Geometry check sheet. Reference: the model listing, model coordinates, mm. A direction names the side the tool comes from. Round coordinates to 2 decimals unless told otherwise and drop trailing zeros. Loops run counter-clockwise (first coordinate to the right, second up) from the corner with the lowest first, then second, coordinate; pieces in that order, holes last. Notation, with made-up numbers: (-19.75, 75.25) - (29.25, 75.25) arc R10 ccw to (29.25, 86.25) - close; hole circle Ø3 at (21.25, -2). An arc over 180 degrees is marked (long way). Write item = value, one per line.
```python
from build123d import *

# Parameters (mm, degrees)
SKETCH1_R                            = 10
BOSS_EXTRUDE1_DEPTH                  = 10
SKETCH1_R_2                          = 20
SKETCH1_R_3                          = 15
BOSS_EXTRUDE1_2_DEPTH                = 10
SKETCH1_R_4                          = 40
SKETCH1_R_5                          = 35
BOSS_EXTRUDE1_3_DEPTH                = 10
BOSS_EXTRUDE2_REACH                  = 89.446
BOSS_EXTRUDE2_END_RADIUS             = 35
BOSS_EXTRUDE2_START                  = 30
BOSS_EXTRUDE2_DIRECTION_2_REACH      = 89.446
BOSS_EXTRUDE2_DIRECTION_2_END_RADIUS = 20
CIRPATTERN1_COUNT                    = 12
BOSS_EXTRUDE3_START                  = 9.76079
BOSS_EXTRUDE3_DEPTH                  = 5.23921
CIRPATTERN3_COUNT                    = 3
SKETCH6_R                            = 1
BOSS_EXTRUDE4_DEPTH                  = 1


with BuildPart() as part:
    # Sketch1 → Boss-Extrude1 (new body)
    with BuildSketch(Plane(origin=(0, 0, 0), x_dir=(1, 0, 0), z_dir=(0, 1, 0))):
        with Locations(Location((0, 0, 0), (0, 0, 270))):
            Circle(SKETCH1_R)
    extrude(amount=BOSS_EXTRUDE1_DEPTH)



with BuildPart() as body_2:
    # Sketch1 → Boss-Extrude1 2 (new body)
    with BuildSketch(Plane(origin=(0, 0, 0), x_dir=(1, 0, 0), z_dir=(0, 1, 0))):
        with Locations(Location((0, 0, 0), (0, 0, 270))):
            Circle(SKETCH1_R_2)
        with Locations(Location((0, 0, 0), (0, 0, 270))):
            Circle(SKETCH1_R_3, mode=Mode.SUBTRACT)
    extrude(amount=BOSS_EXTRUDE1_2_DEPTH)


with BuildPart() as body_3:
    # Sketch1 → Boss-Extrude1 3 (new body)
    with BuildSketch(Plane(origin=(0, 0, 0), x_dir=(1, 0, 0), z_dir=(0, 1, 0))):
        with Locations(Location((0, 0, 0), (0, 0, 270))):
            Circle(SKETCH1_R_4)
        with Locations(Location((0, 0, 0), (0, 0, 270))):
            Circle(SKETCH1_R_5, mode=Mode.SUBTRACT)
    extrude(amount=BOSS_EXTRUDE1_3_DEPTH)


    add(body_2.part)  # Boss-Extrude2 merges body 2
    # Boss-Extrude2: up to this cylinder (the profile starts inside it)
    boss_extrude2_end = Plane(origin=(0, 5, 0), z_dir=(0, -1, 0)) * Cylinder(BOSS_EXTRUDE2_END_RADIUS, 249.892, mode=Mode.PRIVATE)
    # Sketch4 → Boss-Extrude2 (add, up to the surface)
    with BuildSketch(Plane(origin=(0, 0, 0), x_dir=(0, 0, -1), z_dir=(1, 0, 0)).offset(BOSS_EXTRUDE2_START), mode=Mode.PRIVATE) as boss_extrude2_sk1:
        Polygon((-4.262410526, 0), (4.031443844, 10), (5.315133993, 10), (-2.978720377, 0), align=None)
    boss_extrude2_tool1 = extrude(boss_extrude2_sk1.sketch, amount=BOSS_EXTRUDE2_REACH, mode=Mode.PRIVATE) & boss_extrude2_end
    boss_extrude2 = boss_extrude2_tool1.solids().sort_by_distance((30, 5, -0.526362))[0]
    add(boss_extrude2)

    # Boss-Extrude2 direction 2: up to this cylinder (the profile starts outside it)
    boss_extrude2_direction_2_end = Plane(origin=(0, 5, 0), z_dir=(0, -1, 0)) * Cylinder(BOSS_EXTRUDE2_DIRECTION_2_END_RADIUS, 219.892, mode=Mode.PRIVATE)
    # Sketch4 → Boss-Extrude2 direction 2 (add, up to the surface)
    with BuildSketch(Plane(origin=(0, 0, 0), x_dir=(0, 0, -1), z_dir=(1, 0, 0)).offset(BOSS_EXTRUDE2_START), mode=Mode.PRIVATE) as boss_extrude2_direction_2_sk1:
        Polygon((-4.262410526, 0), (4.031443844, 10), (5.315133993, 10), (-2.978720377, 0), align=None)
    boss_extrude2_direction_2_tool1 = extrude(boss_extrude2_direction_2_sk1.sketch, amount=-BOSS_EXTRUDE2_DIRECTION_2_REACH, mode=Mode.PRIVATE) - boss_extrude2_direction_2_end
    boss_extrude2_direction_2 = boss_extrude2_direction_2_tool1.solids().sort_by_distance((30, 5, -0.526362))[0]
    add(boss_extrude2_direction_2)
    boss_extrude2 = boss_extrude2 + boss_extrude2_direction_2  # both directions under the feature's name, for the pattern or mirror that repeats it

    # CirPattern1: Boss-Extrude2 ×12 about axis
    cirpattern1_axis = Axis((0, 0, 0), (0, 1, 0))
    for i in range(1, CIRPATTERN1_COUNT):
        add(boss_extrude2.rotate(cirpattern1_axis, i * 360 / CIRPATTERN1_COUNT))


with BuildPart() as part_1:
    add(part.part)

    add(body_3.part)  # Boss-Extrude3 merges body 3
    # Sketch5 → Boss-Extrude3 (add)
    with BuildSketch(Plane(origin=(0, 0, 0), x_dir=(0, 0, -1), z_dir=(1, 0, 0)).offset(BOSS_EXTRUDE3_START)):
        Polygon((-2.0524403, 10), (1.416675924, 0), (2.174160553, 0), (-1.428789261, 10), align=None)
    boss_extrude3 = extrude(amount=BOSS_EXTRUDE3_DEPTH)

    # CirPattern3: Boss-Extrude3 ×3 about axis
    cirpattern3_axis = Axis((0, 0, 0), (0, 1, 0))
    for i in range(1, CIRPATTERN3_COUNT):
        add(boss_extrude3.rotate(cirpattern3_axis, i * 360 / CIRPATTERN3_COUNT))

    # Sketch6 → Boss-Extrude4 (add)
    with BuildSketch(Plane(origin=(0, 10, 0), x_dir=(1, 0, 0), z_dir=(0, 1, 0))):
        with Locations(Location((0, 0, 0), (0, 0, 270))):
            Circle(SKETCH6_R)
    extrude(amount=BOSS_EXTRUDE4_DEPTH)


solid = part_1.part
```
(1) Mould release check, pull along X, two halves, no side actions. Record for faces 1 (the flat face through (22.8, 5.07, -14.58)), 2 (the flat face through (-8, 10, -1)), 3 (the flat face through (-5.88, 5.07, -10.87)), 4 (the cylindrical face through (-0.976, 10.493, -0.217)): pulls with the +X half, pulls with the -X half, needs draft (parallel to the pull), parting line crosses it, or undercut.
Answers follow:
face_1 = undercut
face_2 = needs draft
face_3 = undercut
face_4 = parting line crosses it
(2) Section check B-B (x = 0). State how many separate pieces and enclosed holes the cut face has, then the cut area to 3 significant figures.
Answers follow:
separate_pieces = 3
enclosed_holes = 0
area = 448 mm²
(3) Section check A-A (x = 11). Enter the section's corners in (y, z), then the cut area to 3 significant figures.
Answers follow:
outline = (0, -38.46) - (10, -38.46) - (10, -33.23) - (0, -33.23) - close; (0, -16.7) - (2.18, -16.7) - (10, -29.68) - (10, -27.12) - (3.72, -16.7) - (10, -16.7) - (10, -10.2) - (0, -10.2) - close; (0, -2.17) - (10, 1.43) - (10, 2.05) - (0, -1.42) - close; (0, 10.2) - (10, 10.2) - (10, 16.7) - (6.56, 16.7) - (0, 27.58) - (0, 25.01) - (5.01, 16.7) - (0, 16.7) - close; (0, 33.23) - (10, 33.23) - (10, 38.46) - (0, 38.46) - close
area = 275 mm²
(4) Gauge pin test, flat ends, axial feed: pin 1 (1.5 mm diameter, centred on x = 10, y = 2, fed in from +Z); pin 2 (2 mm diameter, centred on y = 2, z = -29, fed in from +X); pin 3 (6 mm diameter, centred on x = 22, z = -7, fed in from +Y). Record the tip position at first contact, or that the pin passes through.
Answers follow:
pin_1 = 38.92
pin_2 = 28.57
pin_3 = 10
(5) Set-up check for faces 5 (the flat face through (-6.475, 5.07, 10.53)), 6 (the cylindrical face through (-9.398, 4.93, -33.715)), 7 (the flat face through (-5.83, 4.93, 10.89)): record each of +Z, -Z, +X, -X, +Y, -Y from which the full face is reachable in a straight line by a thin tool's end or side.
Answers follow:
face_5 = -Y
face_6 = none
face_7 = +Y
(6) Section check D-D (x = 25.5). Enter the section's corners in (y, z).
Answers follow:
outline = (0, -30.82) - (10, -30.82) - (10, -23.97) - (0, -23.97) - close; (0, -11.28) - (10, -20.86) - (10, -19.38) - (0, -9.8) - close; (0, 2.98) - (10, -5.32) - (10, -4.03) - (0, 4.26) - close; (0, 18.16) - (10, 8.59) - (10, 10.07) - (0, 19.64) - close; (0, 23.97) - (10, 23.97) - (10, 30.82) - (0, 30.82) - close
(7) Scan lines: L1, parallel to Z at x = 0.5, y = 8; L2, parallel to Z at x = -17, y = 5.25; L3, parallel to X at y = 5.75, z = 8. Record each from-to range of solid material in increasing order. Write a range as [from, to].
Answers follow:
L1 = [-40, -35], [-19.99, -14.99], [-9.99, 9.99], [14.99, 19.99], [35, 40]
L2 = [-36.21, -30.59], [-29.26, -26.69], [-10.54, 11.4], [29.63, 36.21]
L3 = [-39.19, -34.07], [-18.33, -12.69], [-6, 6], [12.69, 18.33], [34.07, 39.19]
